Verification items for the finished model (mm, model axes). Face numbers are marked on the shaded views. A direction names the side the tool comes from. Coordinates: 2 decimals unless noted, no trailing zeros. Write each loop counter-clockwise with the first axis right and the second up, starting at its lowest first coordinate (ties: lowest second). Pieces come first, ordered by that corner, then holes.
```python
from build123d import *

# Parameters (mm, degrees)
SKETCH_1_W          = 25.1
SKETCH_1_H          = 16.1
SKETCH_1_W_2        = 1.9
SKETCH_1_H_2        = 0.6
EXTRUDE_1_DEPTH     = 4.5
SKETCH_2_W          = 1.9
SKETCH_2_H          = 0.6
CUT_EXTRUDE_1_DEPTH = 2
SKETCH_3_W          = 4
SKETCH_3_H          = 16.1
CUT_EXTRUDE_2_DEPTH = 2.8


with BuildPart() as part:
    # 草图1 → 凸台-拉伸1 (new body)
    with BuildSketch(Plane.XY):
        Rectangle(SKETCH_1_W, SKETCH_1_H)
        with Locations((7.4, 8.35)):
            Rectangle(SKETCH_1_W_2, SKETCH_1_H_2)
    extrude(amount=EXTRUDE_1_DEPTH)

    # 草图2 → 切除-拉伸1 (cut)
    with BuildSketch(Plane(origin=(0, 0, 0), x_dir=(-1, 0, 0), z_dir=(0, 0, -1))):
        with Locations((-7.4, 8.35)):
            Rectangle(SKETCH_2_W, SKETCH_2_H)
    extrude(amount=-CUT_EXTRUDE_1_DEPTH, mode=Mode.SUBTRACT)

    # 草图3 → 切除-拉伸2 (cut)
    with BuildSketch(Plane.XY.offset(4.5)):
        with Locations((-10.55, 0)):
            Rectangle(SKETCH_3_W, SKETCH_3_H)
    extrude(amount=-CUT_EXTRUDE_2_DEPTH, mode=Mode.SUBTRACT)


solid = part.part
```
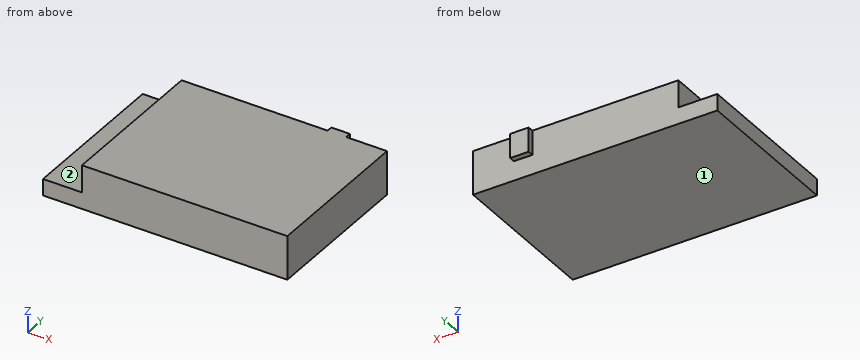
1. Sectioned sample at C-C, the plane x = 7.5. Record the boundary of the cut face in (y, z), and give its area (4 significant figures).
2. Tool access check on the marked faces 1 and 2. Record the directions out of +Z, -Z, +X, -X, +Y, -Y that give a thin tool (end or side, any length) a straight path to the whole face; none if there is none.
3. Sectioned sample at D-D, the plane x = -1.75. Record the boundary of the cut face in (y, z).
4. Gauge pin test, flat ends, axial feed: P1, Ø2, axis at x = 3.5, z = 1.5, coming from the +Y side; P2, Ø0.5, axis at y = 8.5, z = 4, coming from the +X side; P3, Ø1.5, axis at y = 4, z = 3.5, coming from the -X side. Record the tip position at first contact, or that the pin passes through.
5. Sectioned sample at A-A, the plane z = 2.8. Record the boundary of the cut face in (x, y), and give its area (3 significant figures).
6. Material ranges on L1, parallel to X at y = -7, z = 3.1; L2, parallel to Z at x = -9.5, y = -1.5; L3, parallel to Y at x = 6.25, z = 1.6, recorded low to high.
7. Sectioned sample at B-B, the plane y = -2.25. Record the boundary of the cut face in (x, z).
Outcome:
1. outline: (-8.05, 0) - (8.05, 0) - (8.05, 2) - (8.65, 2) - (8.65, 4.5) - (-8.05, 4.5) - close
1. area: 73.95 mm2
2. face 1: -Z, +X, -X, +Y, -Y
2. face 2: +Z, -X, +Y, -Y
3. outline: (-8.05, 0) - (8.05, 0) - (8.05, 4.5) - (-8.05, 4.5) - close
4. P1: stops at y = 8.05
4. P2: stops at x = 8.35
4. P3: stops at x = -8.55
5. outline: (-8.55, -8.05) - (12.55, -8.05) - (12.55, 8.05) - (8.35, 8.05) - (8.35, 8.65) - (6.45, 8.65) - (6.45, 8.05) - (-8.55, 8.05) - close
5. area: 341 mm2
6. L1: x = -8.55 to 12.55
6. L2: z = 0 to 1.7
6. L3: y = -8.05 to 8.05
7. outline: (-12.55, 0) - (12.55, 0) - (12.55, 4.5) - (-8.55, 4.5) - (-8.55, 1.7) - (-12.55, 1.7) - close
